Print and shaded views of the part. All mm, measured from the part's lowest x, y and z. A direction names the side the tool comes from. Give positions to 0.01 mm unless a question says otherwise; leave off trailing zeros. Loops run counter-clockwise (first coordinate to the right, second up) from the corner with the lowest first, then second, coordinate; pieces in that order, holes last. Notation, with made-up numbers: (-1, 59) -> (47, 59) arc R14 cw to (47, 78) -> close; hole circle Ø3 at (26.25, 55). An arc over 180 degrees is marked (long way). Answer as a JSON object with one key per item and string values. Group by question number.
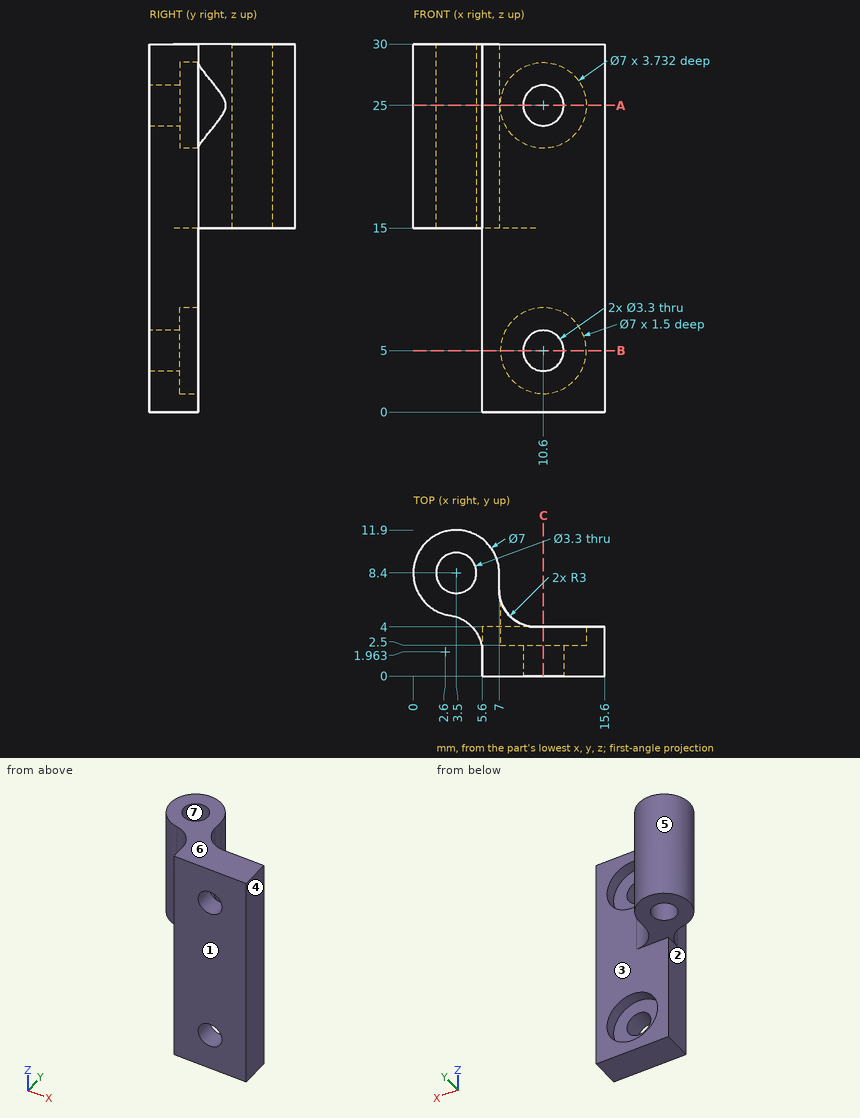
(1) Probe line 1 along Z through (x, y) = (8.25, 2.75) (1 decimal); line 2 along X through (y, z) = (2, 15); line 3 along Y through (x, z) = (6, 9.5). List the from-to ranges inside material, lowest first. Write a range as [from, to].
(2) Pull direction X, two halves, no side cores. Call the marked faces 4, 5, 6 and 7: pulls with the +X half, pulls with the -X half, needs draft (parallel to the pull), parting line crosses it, or undercut.
(3) Saw through at C-C on x = 10.6. List the corners of the cut face in (y, z).
(4) Saw through at A-A on z = 25. Give the number of separate pieces and of enclosed holes in the cut face.
(5) 3-axis set-ups, long thin cutter, end or side, ignore diameter. For the marked faces 1, 2 and 3: which of +Z, -Z, +X, -X, +Y, -Y reach the whole face in a straight line?
(6) Pin check, flat tips, straight feed: pin 1 (3 mm diameter, centred on y = 7, z = 22.5, fed in from -X); pin 2 (5.5 mm diameter, centred on x = 10.5, z = 4, fed in from +Y); pin 3 (4.5 mm diameter, centred on y = 1, z = 15, fed in from -X); pin 4 (2 mm diameter, centred on x = 10.5, z = 26.5, fed in from +Y). Stop position of each tip, or through.
(7) Saw through at B-B on z = 5. List the corners of the cut face in (x, y).
Calculated:
{
 "1": {"line 1": "z = [0, 2.4], [7.6, 22.4], [27.6, 30]", "line 2": "x = [5.6, 15.6]", "line 3": "y = [0, 4]"},
 "2": {"face 4": "pulls with the +X half", "face 5": "parting line crosses it", "face 6": "needs draft", "face 7": "undercut"},
 "3": {"outline": "(0, 0) -> (4, 0) -> (4, 1.5) -> (2.5, 1.5) -> (2.5, 3.35) -> (0, 3.35) -> close; (0, 6.65) -> (2.5, 6.65) -> (2.5, 8.5) -> (4, 8.5) -> (4, 21.5) -> (2.5, 21.5) -> (2.5, 23.35) -> (0, 23.35) -> close; (0, 26.65) -> (2.5, 26.65) -> (2.5, 28.5) -> (4, 28.5) -> (4, 30) -> (0, 30) -> close"},
 "4": {"separate pieces": "2", "enclosed holes": "1"},
 "5": {"face 1": "+Z, -Z, +X, -X, -Y", "face 2": "-Z, -X, -Y", "face 3": "-Z, +X, +Y"},
 "6": {"pin 1": "stops at x = 0", "pin 2": "stops at y = 4", "pin 3": "stops at x = 5.31", "pin 4": "stops at y = 2.5"},
 "7": {"outline": "(5.6, 0) -> (8.95, 0) -> (8.95, 2.5) -> (7.1, 2.5) -> (7.1, 4) -> (5.6, 4) -> close; (12.25, 0) -> (15.6, 0) -> (15.6, 4) -> (14.1, 4) -> (14.1, 2.5) -> (12.25, 2.5) -> close"}
}
